from build123d import *

# Parameters (mm, degrees)
F1_DEPTH = 63.5
F2_DEPTH = 25.4
F3_DEPTH = 7.9375
F0_W     = 36.734618
F0_H     = 28.575
F5_R     = 6.35


with BuildPart() as f1:
    # F0 (on Front) → F1 (new body, symmetric)
    with BuildSketch(Plane.XZ):
        Polygon((-41.275, 9.525), (-41.275, -9.525), (41.275, -9.525), (41.275, 9.525), (22.225, 9.525), align=None)
    extrude(amount=F1_DEPTH, both=True)

    # F0 (on Front) → F2 (join, symmetric)
    with BuildSketch(Plane.XZ):
        with BuildLine():
            Line((22.225, 9.525), (41.275, 9.525))
            Line((41.275, 9.525), (41.275, 27.0002))
            ThreePointArc((41.275, 27.0002), (45.92468, 38.22552), (57.15, 42.8752))
            Line((57.15, 42.8752), (60.325, 42.8752))
            Line((60.325, 42.8752), (60.325, 61.9252))
            Line((60.325, 61.9252), (57.15, 61.9252))
            add(Edge.make_bspline(
                [(50.826813, 61.348023), (52.907758, 61.552865), (55.015741, 61.744854), (57.15, 61.9252)],
                knots=[106.970225, 106.970225, 106.970225, 106.970225, 111.504536, 111.504536, 111.504536, 111.504536], degree=3))
            ThreePointArc((50.826813, 61.348023), (30.311661, 49.348783), (22.225, 27.0002))
            Line((22.225, 27.0002), (22.225, 9.525))
        make_face()
        Polygon((60.325, 66.675), (60.325, 61.9252), (60.325, 42.8752), (60.325, 38.1), (74.390382, 38.1), (74.390382, 66.675), align=None)
    extrude(amount=F2_DEPTH, both=True)

    # F0 (on Front) → F3 (join, symmetric)
    with BuildSketch(Plane.XZ):
        with BuildLine():
            add(Edge.make_bspline(
                [(-41.275, 9.525), (-32.308794, 44.530056), (1.734671, 56.515538), (50.826813, 61.348023)],
                knots=[0, 0, 0, 0, 106.970225, 106.970225, 106.970225, 106.970225], degree=3))
            Line((-41.275, 9.525), (22.225, 9.525))
            Line((22.225, 9.525), (22.225, 27.0002))
            ThreePointArc((22.225, 27.0002), (30.311661, 49.348783), (50.826813, 61.348023))
        make_face()
    extrude(amount=F3_DEPTH, both=True)

    # F0 (on Front) → F4 (revolve)
    with BuildSketch(Plane.XZ):
        with Locations((92.757691, 52.3875)):
            Rectangle(F0_W, F0_H)
    revolve(axis=Axis((74.390382, 0, 52.3875), (0, 0, 1)))

    # F5
    f5_edges = [f1.edges().sort_by_distance(p)[0] for p in [
        (-41.275, -63.5, 0),
        (41.275, -63.5, 0),
        (41.275, 63.5, 0),
        (-41.275, 63.5, 0),
    ]]
    fillet(f5_edges, radius=F5_R)


solid = f1.part
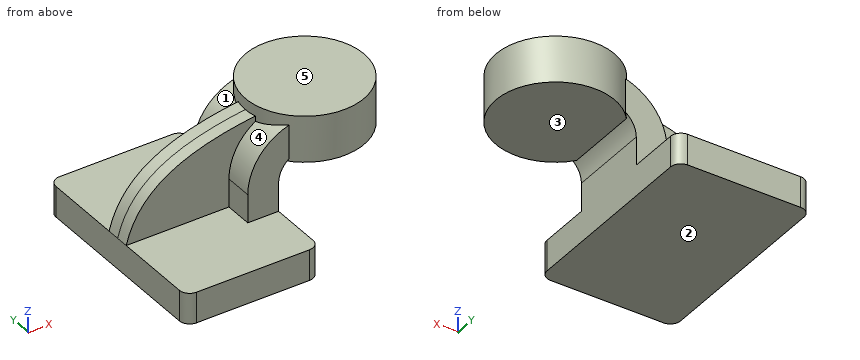
Geometry: final body of the model. Coordinates: model frame, mm. Face numbers are marked on the shaded views. A direction names the side the tool comes from. Coordinates: 2 decimals unless noted, no trailing zeros. Loops run counter-clockwise (first coordinate to the right, second up) from the corner with the lowest first, then second, coordinate; pieces in that order, holes last. Notation, with made-up numbers: (32, 80) - (72, 80) arc R15 ccw to (72, 109) - close; hole circle Ø5 at (27.5, 34). An arc over 180 degrees is marked (long way). Put each result on its own line as item: value. Start each with the question number.
Q1. Set-up query: the marked faces 1, 2, 3, 4 and 5. Return all of +Z, -Z, +X, -X, +Y, -Y with unobstructed straight access to the full face (end or side cutting, diameter ignored); none if empty.
Q2. Cut plane A-A, the plane z = 0. Return loops of the section in (x, y) (3 decimals).
Q3. Cut plane B-B, the plane y = 16.5. Return loops of the section in (x, z) (3 decimals).
Q4. Cut plane C-C, the plane x = 72. Return loops of the section in (y, z) (3 decimals).
Q5. Pin query (flat end, axial travel): pin 1 Ø2 at (x, z) = (-2.5, 31.5) entering from -Y; pin 2 Ø1.5 at (x, z) = (41, 16) entering from +Y; pin 3 Ø5 at (y, z) = (-19, 16) entering from -X (3 decimals). Return the tip coordinate at first contact, or that it passes through.
Q6. Line query: line 1 (Z direction, x = 47, y = 10) (3 decimals); line 2 (X direction, y = -3.5, z = 2.5) (3 decimals); line 3 (Z direction, x = -34, y = 34) (3 decimals). Output: solid intervals per line, ascending.
Filled sheet:
1. face 1: +Z, -X, +Y
1. face 2: -Z, +X, -X, +Y, -Y
1. face 3: -Z, +X, +Y, -Y
1. face 4: +Z, -X, -Y
1. face 5: +Z, +X, -X, +Y, -Y
2. outline: (-41.275, -57.15) arc R6.35 ccw to (-34.925, -63.5) - (34.925, -63.5) arc R6.35 ccw to (41.275, -57.15) - (41.275, 57.15) arc R6.35 ccw to (34.925, 63.5) - (-34.925, 63.5) arc R6.35 ccw to (-41.275, 57.15) - close
3. outline: (-41.275, -9.525) - (41.275, -9.525) - (41.275, 27) arc R15.875 cw to (45.801, 38.1) - (107.211, 38.1) - (107.211, 66.675) - (41.57, 66.675) - (41.57, 58.257) arc R34.925 ccw to (22.225, 27) - (22.225, 9.525) - (-41.275, 9.525) - close
4. outline: (-36.657, 38.1) - (36.657, 38.1) - (36.657, 66.675) - (-36.657, 66.675) - close
5. pin 1: y = -7.94
5. pin 2: y = 25.4
5. pin 3: x = 22.225
6. line 1: 38.1 to 66.675
6. line 2: -41.275 to 41.275
6. line 3: -9.525 to 9.525
